The listing builds one solid part. Answer for the finished solid, in the listing's coordinates (mm). A direction names the side the tool comes from. Coordinates: 2 decimals unless noted, no trailing zeros. Write each loop counter-clockwise with the first axis right and the second up, starting at its lowest first coordinate (ties: lowest second). Pieces come first, ordered by that corner, then holes.
from build123d import *

# Parameters (mm, degrees)
SKETCH1_R           = 3.4
SKETCH1_R_2         = 2.1
BOSS_EXTRUDE1_DEPTH = 100


with BuildPart() as part:
    # Sketch1 → Boss-Extrude1 (new body)
    with BuildSketch(Plane(origin=(0, 0, 0), x_dir=(0, 0, -1), z_dir=(1, 0, 0))):
        with BuildLine():
            Line((-15, 1.7), (-15, -13))
            ThreePointArc((-15, -13), (-14.414213562, -14.414213562), (-13, -15))
            Line((-13, -15), (-4.3, -15))
            ThreePointArc((-4.3, -15), (-4.087867966, -14.912132034), (-4, -14.7))
            Line((-4, -14.7), (-4, -13))
            Line((-4, -13), (-8.25, -13))
            Line((-8.25, -13), (-8.25, -9.664213562))
            Line((-8.25, -9.664213562), (-4.585786438, -6))
            Line((-4.585786438, -6), (4.585786438, -6))
            Line((4.585786438, -6), (8.25, -9.664213562))
            Line((8.25, -9.664213562), (8.25, -13))
            Line((8.25, -13), (4, -13))
            Line((4, -13), (4, -14.7))
            ThreePointArc((4, -14.7), (4.087867966, -14.912132034), (4.3, -15))
            Line((4.3, -15), (13, -15))
            ThreePointArc((13, -15), (14.414213562, -14.414213562), (15, -13))
            Line((15, -13), (15, 1.7))
            ThreePointArc((15, 1.7), (14.912132034, 1.912132034), (14.7, 2))
            Line((14.7, 2), (13, 2))
            Line((13, 2), (13, -1))
            Line((13, -1), (12, -1))
            Line((12, -1), (9, 2))
            Line((9, 2), (9, 8))
            Line((9, 8), (12, 11))
            Line((12, 11), (13, 11))
            Line((13, 11), (13, 8))
            Line((13, 8), (14.7, 8))
            ThreePointArc((14.7, 8), (14.912132034, 8.087867966), (15, 8.3))
            Line((15, 8.3), (15, 13))
            ThreePointArc((15, 13), (14.414213562, 14.414213562), (13, 15))
            Line((13, 15), (4.3, 15))
            ThreePointArc((4.3, 15), (4.087867966, 14.912132034), (4, 14.7))
            Line((4, 14.7), (4, 13))
            Line((4, 13), (8.25, 13))
            Line((8.25, 13), (8.25, 9.664213562))
            Line((8.25, 9.664213562), (4.585786438, 6))
            Line((4.585786438, 6), (-4.585786438, 6))
            Line((-4.585786438, 6), (-8.25, 9.664213562))
            Line((-8.25, 9.664213562), (-8.25, 13))
            Line((-8.25, 13), (-4, 13))
            Line((-4, 13), (-4, 14.7))
            ThreePointArc((-4, 14.7), (-4.087867966, 14.912132034), (-4.3, 15))
            Line((-4.3, 15), (-13, 15))
            ThreePointArc((-13, 15), (-14.414213562, 14.414213562), (-15, 13))
            Line((-15, 13), (-15, 8.3))
            ThreePointArc((-15, 8.3), (-14.912132034, 8.087867966), (-14.7, 8))
            Line((-14.7, 8), (-13, 8))
            Line((-13, 8), (-13, 11))
            Line((-13, 11), (-12, 11))
            Line((-12, 11), (-9, 8))
            Line((-9, 8), (-9, 2))
            Line((-9, 2), (-12, -1))
            Line((-12, -1), (-13, -1))
            Line((-13, -1), (-13, 2))
            Line((-13, 2), (-14.7, 2))
            ThreePointArc((-14.7, 2), (-14.912132034, 1.912132034), (-15, 1.7))
        make_face()
        Circle(SKETCH1_R, mode=Mode.SUBTRACT)
        with Locations((-11.625, -11.625)):
            Circle(SKETCH1_R_2, mode=Mode.SUBTRACT)
        with Locations((11.625, -11.625)):
            Circle(SKETCH1_R_2, mode=Mode.SUBTRACT)
        Polygon((-13, -2.5), (-13, -8.25), (-9.664213562, -8.25), (-6, -4.585786438), (-6, 2), (-6.878679656, 2), (-11.378679656, -2.5), align=None, mode=Mode.SUBTRACT)
        Polygon((6, 2), (6, -4.585786438), (9.664213562, -8.25), (13, -8.25), (13, -2.5), (11.378679656, -2.5), (6.878679656, 2), align=None, mode=Mode.SUBTRACT)
    extrude(amount=BOSS_EXTRUDE1_DEPTH)


solid = part.part
Q1. Given pin 1 (1.9 mm diameter, centred on x = 55, y = -14, fed in from -Z); pin 2 (1.4 mm diameter, centred on x = 34, z = 14, fed in from -Y); pin 3 (1.4 mm diameter, centred on x = 25.5, z = 14, fed in from +Y); pin 4 (0.8 mm diameter, centred on x = 35.5, y = -13.5, fed in from +Z), each flat-ended and moving along its own axis, determine where each tip first touches the part or whether it passes through.
Answers below:
pin 1: stops at z = -15
pin 2: stops at y = -14.98
pin 3: stops at y = 14.98
pin 4: stops at z = 15
Q2. The part is cut by section B-B, the plane y = 0. Write down the section's boundary in (x, z).
Answers below:
outline: (0, -15) - (100, -15) - (100, -13) - (0, -13) - close; (0, -11) - (100, -11) - (100, -8.88) - (0, -8.88) - close; (0, -6) - (100, -6) - (100, -3.4) - (0, -3.4) - close; (0, 3.4) - (100, 3.4) - (100, 6) - (0, 6) - close; (0, 8.88) - (100, 8.88) - (100, 11) - (0, 11) - close; (0, 13) - (100, 13) - (100, 15) - (0, 15) - close
Q3. Determine the mould class of faces 3 (the face through (49, -5, -13)), 4 (the face through (49, 2, 14)), 5 (the face through (49.3, -14.4, 14.43)), 6 (the face through (49, -6, -15)) for opening direction Z: released by +Z, released by -Z, zero draft, split by the parting line, or undercut.
Answers below:
face 3: undercut
face 4: zero draft
face 5: released by +Z
face 6: released by -Z
Q4. Which of the six approach directions +Z, -Z, +X, -X, +Y, -Y give full straight-line access (tool end or side, diameter ignored) to faces 1 (the face through (49, -1, -6)), 2 (the face through (49, -15, -9))?
Answers below:
face 1: +X, -X
face 2: +Z, -Z, +X, -X, -Y
Q5. The part is cut by section C-C, the plane x = 25.5. State how many separate pieces and enclosed holes the cut face has, then the cut area to 3 significant figures.
Answers below:
separate pieces: 1
enclosed holes: 5
area: 399 mm2
Q6. Find the intervals of material crossed by probe 1 along Z at (x, y) = (8, 1.75); probe 2 along Y at (x, z) = (91, 8); probe 3 along Z at (x, y) = (84.5, -12.75), in increasing order.
Answers below:
probe 1: z = -15 to -13, -9.25 to -7.13, -6 to -2.92, 2.92 to 6, 7.13 to 9.25, 13 to 15
probe 2: y = -15 to -13, -9.41 to -6.59, 0.88 to 9.41, 13 to 15
probe 3: z = -15 to -13.4, -9.85 to -8.25, 8.25 to 9.85, 13.4 to 15
Q7. The part is cut by section A-A, the plane z = 0. Write down the section's boundary in (x, y), then the cut area to 3 significant figures.
Answers below:
outline: (0, -6) - (100, -6) - (100, -3.4) - (0, -3.4) - close; (0, 3.4) - (100, 3.4) - (100, 6) - (0, 6) - close
area: 520 mm2
